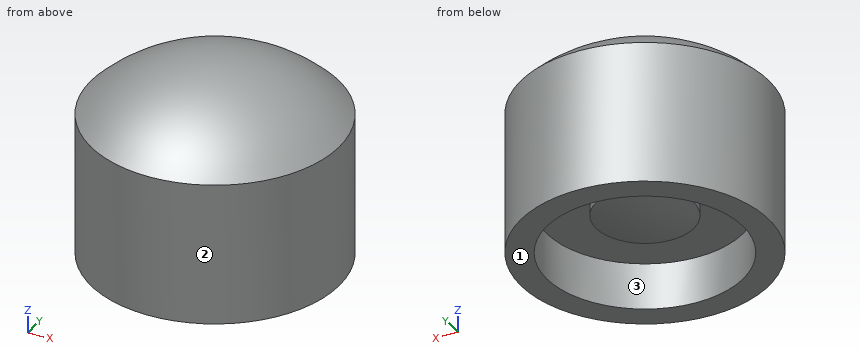
```python
from build123d import *

# Parameters (mm, degrees)
ESBO_O1_R                = 6.95
RESSALTO_EXTRUS_O1_DEPTH = 8
ESBO_O2_R                = 6.5
CORTE_EXTRUS_O1_DEPTH    = 4
ESBO_O3_R                = 5.5
CORTE_EXTRUS_O2_DEPTH    = 11.611550311


with BuildPart() as part:
    # Esboço1 → Ressalto-extrusão1 (new body)
    with BuildSketch(Plane.XY):
        Circle(ESBO_O1_R)
    extrude(amount=RESSALTO_EXTRUS_O1_DEPTH)

    # Esboço2 → Corte-extrusão1 (cut)
    with BuildSketch(Plane.XY.offset(8)):
        Circle(ESBO_O2_R)
    extrude(amount=-CORTE_EXTRUS_O1_DEPTH, mode=Mode.SUBTRACT)

    # Esboço3 → Corte-extrusão2 (cut, through all)
    with BuildSketch(Plane.XY.offset(4)):
        Circle(ESBO_O3_R)
    extrude(amount=-CORTE_EXTRUS_O2_DEPTH, mode=Mode.SUBTRACT)

    # Esboço4 → Revolução1 (revolve)
    with BuildSketch(Plane(origin=(0, 0, 0), x_dir=(1, 0, 0), z_dir=(0, 1, 0))):
        with BuildLine():
            Line((-6.95, -8), (-6.5, -8))
            Line((-6.5, -8), (-6.5, -6.423040188))
            Line((-6.5, -6.423040188), (-4.052357622, -6.423040188))
            ThreePointArc((-4.052357622, -6.423040188), (-2.736736603, -9.045296291), (0, -10.10234809))
            Line((0, -10.10234809), (0, -10.899494937))
            ThreePointArc((0, -10.899494937), (-3.765287867, -10.145558539), (-6.95, -8))
        make_face()
    revolve(axis=Axis((0, 0, 0), (0, 0, 1)))

    # Esboço5 → Revolução2 (revolve)
    with BuildSketch(Plane(origin=(0, 0, 0), x_dir=(1, 0, 0), z_dir=(0, 1, 0)), mode=Mode.PRIVATE) as revolu_o2_sk:
        with BuildLine():
            Line((-3.713977707, -5.421872189), (-3.713977707, -6.04883524))
            ThreePointArc((-3.713977707, -6.04883524), (-1.937414068, -6.871607812), (0, -7.153671279))
            Line((0, -7.153671279), (0, -6.423040188))
            ThreePointArc((0, -6.423040188), (-1.744054919, -5.991033293), (-3.084817583, -4.794909137))
            Line((-3.084817583, -4.794909137), (-3.713977707, -4.794909137))
            Line((-3.713977707, -4.794909137), (-3.713977707, -3.721064783))
            Line((-3.713977707, -3.721064783), (-5.5, -3.721064783))
            Line((-5.5, -3.721064783), (-5.5, -5.421872189))
            Line((-5.5, -5.421872189), (-3.713977707, -5.421872189))
        make_face()
    revolve(revolu_o2_sk.sketch.rotate(Axis((0, 0, 10.899494937), (0, 0, -1)), 180), axis=Axis((0, 0, 10.899494937), (0, 0, -1)))

    # Esboço7 → Revolução3 (revolve)
    with BuildSketch(Plane(origin=(0, 0, 0), x_dir=(1, 0, 0), z_dir=(0, 1, 0)), mode=Mode.PRIVATE) as revolu_o3_sk:
        with BuildLine():
            Line((-2.735445453, -4.263680727), (-2.735445453, -3.250344697))
            Line((-2.735445453, -3.250344697), (-5.5, -3.250344697))
            Line((-5.5, -3.250344697), (-5.5, -2.605717645))
            Line((-5.5, -2.605717645), (-2.735445453, -2.605717645))
            Line((-2.735445453, -2.605717645), (-2.735445453, -2.145225421))
            ThreePointArc((-2.735445453, -2.145225421), (-1.373890676, -1.95031325), (0, -1.885147489))
            Line((0, -1.885147489), (0, -3.721064783))
            ThreePointArc((0, -3.721064783), (-1.394372071, -3.858027591), (-2.735445453, -4.263680727))
        make_face()
    revolve(revolu_o3_sk.sketch.rotate(Axis((0, 0, 10.899494937), (0, 0, -1)), 180), axis=Axis((0, 0, 10.899494937), (0, 0, -1)))


solid = part.part
```
Verification items for the finished model (mm, model axes). Face numbers are marked on the shaded views. Coordinates: 2 decimals unless noted, no trailing zeros. Loops run counter-clockwise (first coordinate to the right, second up) from the corner with the lowest first, then second, coordinate; pieces in that order, holes last. Notation, with made-up numbers: (45, -20.5) -> (75, -20.5) arc R20 ccw to (75, -1.5) -> close; hole circle Ø6 at (-16, 30.25). An arc over 180 degrees is marked (long way). Answer in a Markdown table with one row per item. Add a question column.
1. Section check A-A, the plane z = 4.5. Enter the section's corners in (x, y).
2. Section check B-B, the plane x = 4.25. Enter the section's corners in (y, z), then the cut area to 3 significant figures.
3. Material ranges on probe 1 along Y at (x, z) = (0, 4.6); probe 2 along Z at (x, y) = (-3.5, 0.25); probe 3 along Y at (x, z) = (-1.75, 5.25), recorded low to high. Write a range as [from, to].
4. Draft check along X on the marked faces 1, 2 and 3. Enter one of: +X half, -X half, draft (parallel to the pull), parting line (faces both ways), or undercut.
5. Section check C-C, the plane y = 5.25. Enter the section's corners in (x, z).
6. Section check D-D, the plane y = -6. Enter the section's corners in (x, z), then the cut area to 3 significant figures.
7. Depth check by flat-ended pin: P1, Ø6, axis at x = -0.5, y = 3.5, coming from the +Z side; P2, Ø1.5, axis at x = -3.5, y = -5, coming from the +Z side; P3, Ø8, axis at x = 1, y = 3, coming from the -Z side; P4, Ø1, axis at y = -3, z = 6.5, coming from the +X side. Enter the tip coordinate at first touch or a pass-through.
Derived:
| question | item | result |
|---|---|---|
| 1 | outline | circle Ø13.9 at (0, 0); circle Ø11 at (0, 0); hole circle Ø13 at (0, 0); hole circle Ø7.43 at (0, 0) |
| 2 | outline | (-5.5, 0) -> (-3.49, 0) -> (-3.49, 2.61) -> (3.49, 2.61) -> (3.49, 0) -> (5.5, 0) -> (5.5, 8) arc R8.81 ccw to (-5.5, 8) -> close; hole (-4.92, 4) -> (-3.49, 4) -> (-3.49, 5.42) -> (3.49, 5.42) -> (3.49, 4) -> (4.92, 4) -> (4.92, 6.42) -> (-4.92, 6.42) -> close; hole (-3.49, 3.25) -> (3.49, 3.25) -> (3.49, 3.72) -> (-3.49, 3.72) -> close |
| 2 | area | 67.1 mm² |
| 3 | probe 1 | y = [-6.95, -6.5], [-5.5, -3.71], [3.71, 5.5], [6.5, 6.95] |
| 3 | probe 2 | z = [2.61, 3.25], [4.79, 6.18], [8.1, 10.25] |
| 3 | probe 3 | y = [-6.73, -6.26], [-5.21, -2.08], [2.08, 5.21], [6.26, 6.73] |
| 4 | face 1 | draft |
| 4 | face 2 | parting line |
| 4 | face 3 | undercut |
| 5 | outline | (-4.55, 0) -> (-1.64, 0) -> (-1.64, 2.61) -> (1.64, 2.61) -> (1.64, 0) -> (4.55, 0) -> (4.55, 8) arc R8.25 ccw to (-4.55, 8) -> close; hole (-3.83, 4) -> (-1.64, 4) -> (-1.64, 5.42) -> (1.64, 5.42) -> (1.64, 4) -> (3.83, 4) -> (3.83, 6.42) -> (-3.83, 6.42) -> close; hole (-1.64, 3.25) -> (1.64, 3.25) -> (1.64, 3.72) -> (-1.64, 3.72) -> close |
| 6 | outline | (-3.51, 0) -> (3.51, 0) -> (3.51, 8) arc R7.72 ccw to (-3.51, 8) -> close; hole (-2.5, 4) -> (2.5, 4) -> (2.5, 6.42) -> (-2.5, 6.42) -> close |
| 6 | area | 48.0 mm² |
| 7 | P1 | stops at z = 10.88 |
| 7 | P2 | stops at z = 9.3 |
| 7 | P3 | stops at z = 0 |
| 7 | P4 | stops at x = 6.48 |
